Here's how the part is built. I have some questions about the finished solid (model axes, mm). Face numbers are marked on the shaded views. A direction names the side the tool comes from. Round coordinates to 2 decimals unless told otherwise and drop trailing zeros. Order: outer loops, then holes, each group sorted by start corner. A loop starts at its lowest first (then second) coordinate and runs counter-clockwise, first axis right, second up. Notation, with made-up numbers: M 15,-35 L 57,-35 A32 ccw 57,-8 Z; hole C -16.75,72.25 d3. An arc over 180 degrees is marked long. Answer as CSV lines item,"result". Start each with the question number.
```python
from build123d import *

# Parameters (mm, degrees)
PAD002_DEPTH          = 100
POLARPATTERN001_COUNT = 4
SKETCH_W              = 110
SKETCH_H              = 110
PAD_DEPTH             = 2
SKETCH001_W           = 110
SKETCH001_H           = 110
SKETCH001_W_2         = 106
SKETCH001_H_2         = 106
PAD001_DEPTH          = 140
PAD003_DEPTH          = 20
POLARPATTERN_COUNT    = 4
CHAMFER_SIZE          = 15


with BuildPart() as body001:
    # Sketch003 → Pad002 (new body)
    with BuildSketch(Plane.XZ):
        Polygon((-23, 68.162831), (-23, 101.837169), (0, 108), (23, 101.837169), (23, 68.162831), (0, 62), align=None)
    pad002 = extrude(amount=PAD002_DEPTH)

    # PolarPattern001: Pad002 ×4 about axis
    polarpattern001_axis = Axis((0, 0, 0), (0, 0, 1))
    for i in range(1, POLARPATTERN001_COUNT):
        add(pad002.rotate(polarpattern001_axis, i * 360 / POLARPATTERN001_COUNT))


with BuildPart() as chamfer_body:
    # Sketch → Pad (new body)
    with BuildSketch(Plane.XY):
        Rectangle(SKETCH_W, SKETCH_H)
    extrude(amount=PAD_DEPTH)

    # Sketch001 (on Face6 of Pad) → Pad001 (join)
    with BuildSketch(Plane.XY.offset(2)):
        Rectangle(SKETCH001_W, SKETCH001_H)
        Rectangle(SKETCH001_W_2, SKETCH001_H_2, mode=Mode.SUBTRACT)
    extrude(amount=PAD001_DEPTH)

    # Sketch002 (on Face10 of Pad001) → Pad003 (join)
    with BuildSketch(Plane.XZ.offset(55)):
        Polygon((-25, 66.69873), (0, 60), (25, 66.69873), (25, 103.30127), (0, 110), (-25, 103.30127), align=None)
    pad003 = extrude(amount=PAD003_DEPTH)

    # PolarPattern: Pad003 ×4 about axis
    polarpattern_axis = Axis((0, 0, 0), (0, 0, 1))
    for i in range(1, POLARPATTERN_COUNT):
        add(pad003.rotate(polarpattern_axis, i * 360 / POLARPATTERN_COUNT))

    # Cut: cut Body001
    add(body001.part, mode=Mode.SUBTRACT)

    # Chamfer
    chamfer_edges = [chamfer_body.edges().sort_by_distance(p)[0] for p in [
        (-55, 55, 1),
        (55, 55, 1),
        (-55, -55, 1),
        (55, -55, 1),
        (-55, 55, 72),
        (55, 55, 72),
        (-55, -55, 72),
        (55, -55, 72),
        (-53, 53, 72),
        (53, 53, 72),
        (53, -53, 72),
        (-53, -53, 72),
    ]]
    chamfer(chamfer_edges, length=CHAMFER_SIZE)


solid = chamfer_body.part
```
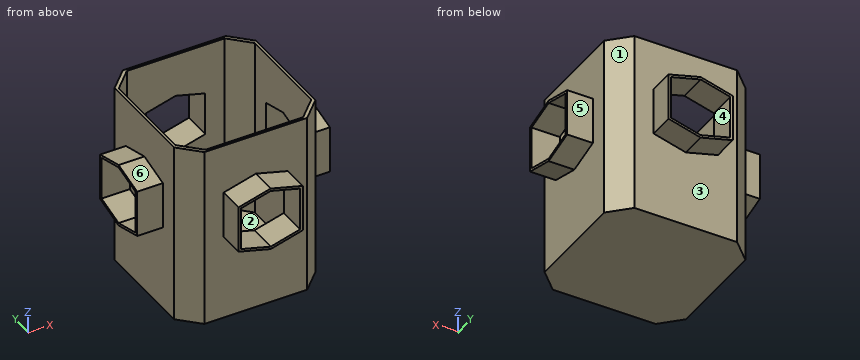
Item 1: Which directions (+Z, -Z, +X, -X, +Y, -Y) give clear straight access to the entire face, cutting with the end or side of a thin tool? Please do the marked faces 4, 5 and 6.
Item 2: For P1, Ø8, axis at x = -7, z = 16, coming from the +Y side; P2, Ø10, axis at y = 69.5, z = 92, coming from the -X side; P3, Ø12, axis at x = -5.5, y = -45, coming from the +Z side, each with a flat end and sliding along its axis, tell me the tip position at first contact or that it passes through.
Item 3: We'd pull the mould along X, two halves only. Please class the marked faces 1, 2 and 3: pulls with the +X half, pulls with the -X half, needs draft (parallel to the pull), parting line crosses it, or undercut.
Item 4: If I drill on line 1 along Y through (x, z) = (-61, 71); line 2 along Y through (x, z) = (-33.5, 131), over which ranges is the centre line in solid material (lowest first)?
Item 5: If we section it at B-B on y = 50: Please give me the cut outline in (x, z), and give its area (3 significant figures).
Item 6: If we section it at C-C on z = 31.5: Please give me the cut outline in (x, y).
Item 7: If we section it at A-A on x = -10: Please give me the cut outline in (y, z).
Item 8: If we section it at D-D on x = 59: Please give me the cut outline in (y, z), and give its area (3 significant figures).
Geometry says:
1,face 4,"+Y, -Y"
1,face 5,"+Z, -Z, +X, +Y"
1,face 6,"+Z, -X, -Y"
2,P1,"y = 55"
2,P2,"x = -25"
2,P3,"z = 2"
3,face 1,"pulls with the +X half"
3,face 2,"undercut"
3,face 3,"needs draft"
4,line 1,"-25 to -23, 23 to 25"
4,line 2,"-55 to -53, 53 to 55"
5,outline,"M -45,0 L 45,0 L 45,142 L 41,142 L 41,2 L -41,2 L -41,142 L -45,142 Z"
5,area,"1,300 mm²"
6,outline,"M -55,-40 L -40,-55 L 40,-55 L 55,-40 L 55,40 L 40,55 L -40,55 L -55,40 Z; hole M -53,-38 L -38,-53 L 38,-53 L 53,-38 L 53,38 L 38,53 L -38,53 L -53,38 Z"
7,outline,"M -75,62.68 L -55,62.68 L -55,0 L 55,0 L 55,62.68 L 75,62.68 L 75,64.68 L 53,64.68 L 53,2 L -53,2 L -53,64.68 L -75,64.68 Z; M -75,105.32 L -53,105.32 L -53,142 L -55,142 L -55,107.32 L -75,107.32 Z; M 53,105.32 L 75,105.32 L 75,107.32 L 55,107.32 L 55,142 L 53,142 Z"
8,outline,"M -25,66.7 L 0,60 L 25,66.7 L 25,103.3 L 0,110 L -25,103.3 Z; hole M -23,68.16 L 0,62 L 23,68.16 L 23,101.84 L 0,108 L -23,101.84 Z"
8,area,"333 mm²"
